CAD build for the part. Positions are in the model's coordinates, mm. A direction names the side the tool comes from. Round coordinates to 2 decimals unless told otherwise and drop trailing zeros. Write each loop counter-clockwise with the first axis right and the second up, starting at its lowest first coordinate (ties: lowest second). Pieces come first, ordered by that corner, then holes. Notation, with made-up numbers: (18, -39) -> (55, -39) arc R16 ccw to (55, -11) -> close; hole circle Ø4 at (43.25, 39). An arc over 180 degrees is marked (long way). Answer in a Markdown table with one row per item. Add a question column.
```python
from build123d import *

# Parameters (mm, degrees)
SKETCH_1_W                   = 30
SKETCH_1_H                   = 35
EXTRUDE_1_DEPTH              = 10.5
CUT_EXTRUDE_1_DEPTH          = 8
FILLET_1_R                   = 1
HOLE_WIZARD_M2_1_D           = 2.1
HOLE_WIZARD_M2_1_DEPTH       = 20
HOLE_WIZARD_M2_1_CBORE_D     = 4.2
HOLE_WIZARD_M2_1_CBORE_DEPTH = 2
HOLE_WIZARD_M2_1_TIP         = 0.63090365


with BuildPart() as part:
    # ｽｹｯﾁ1 → ﾎﾞｽ - 押し出し1 (new body)
    with BuildSketch(Plane(origin=(0, 0, 0), x_dir=(1, 0, 0), z_dir=(0, 1, 0))):
        Rectangle(SKETCH_1_W, SKETCH_1_H)
    extrude(amount=EXTRUDE_1_DEPTH)

    # ｽｹｯﾁ2 → ｶｯﾄ - 押し出し1 (cut)
    with BuildSketch(Plane(origin=(0, 10.5, 0), x_dir=(1, 0, 0), z_dir=(0, 1, 0))):
        with BuildLine():
            Line((15, 12.5), (15, -12.5))
            Line((15, -12.5), (12.5, -12.5))
            ThreePointArc((12.5, -12.5), (10.732233047, -13.232233047), (10, -15))
            Line((10, -15), (10, -17.5))
            Line((10, -17.5), (12.5, -17.5))
            Line((12.5, -17.5), (17, -17.5))
            Line((17, -17.5), (17, 17.5))
            Line((17, 17.5), (12.5, 17.5))
            Line((12.5, 17.5), (10, 17.5))
            Line((10, 17.5), (10, 15))
            ThreePointArc((10, 15), (10.732233047, 13.232233047), (12.5, 12.5))
            Line((12.5, 12.5), (15, 12.5))
        make_face()
    cut_extrude_1 = extrude(amount=-CUT_EXTRUDE_1_DEPTH, mode=Mode.SUBTRACT)

    # ﾐﾗｰ1: ｶｯﾄ - 押し出し1 across plane
    add(cut_extrude_1.mirror(Plane(origin=(0, 0, 0), x_dir=(0, 0, 1), z_dir=(1, 0, 0))), mode=Mode.SUBTRACT)

    # ﾌｨﾚｯﾄ1
    fillet_1_edges = [part.edges().sort_by_distance(p)[0] for p in [
        (15, 10.5, 0),
        (0, 10.5, -17.5),
        (15, 1.25, 17.5),
        (15, 1.25, -17.5),
        (13.75, 10.5, 12.5),
        (10.732233047, 10.5, 13.232233047),
        (10, 10.5, 16.25),
        (13.75, 10.5, -12.5),
        (10, 10.5, -16.25),
        (10.732233047, 10.5, -13.232233047),
        (10, 6.5, -17.5),
        (10, 6.5, 17.5),
        (15, 6.5, 12.5),
        (15, 6.5, -12.5),
        (-15, 10.5, 0),
        (0, 10.5, 17.5),
        (-15, 1.25, 17.5),
        (-15, 1.25, -17.5),
        (-10, 6.5, 17.5),
        (-10.732233047, 10.5, -13.232233047),
        (-13.75, 10.5, -12.5),
        (-15, 6.5, -12.5),
        (-13.75, 10.5, 12.5),
        (-15, 6.5, 12.5),
        (-10.732233047, 10.5, 13.232233047),
        (-10, 10.5, 16.25),
        (-10, 10.5, -16.25),
        (-10, 6.5, -17.5),
    ]]
    fillet(fillet_1_edges, radius=FILLET_1_R)

    # M2 なべ頭ねじ用座ぐり穴1
    with Locations(Plane(origin=(0, 2.5, 0), x_dir=(1, 0, 0), z_dir=(0, 1, 0))):
        with Locations((12.5, -15), (12.5, 15), (-12.5, 15), (-12.5, -15)):
            CounterBoreHole(HOLE_WIZARD_M2_1_D / 2, HOLE_WIZARD_M2_1_CBORE_D / 2, HOLE_WIZARD_M2_1_CBORE_DEPTH, depth=HOLE_WIZARD_M2_1_DEPTH)
            with Locations((0, 0, -(HOLE_WIZARD_M2_1_DEPTH + HOLE_WIZARD_M2_1_TIP / 2))):  # 118° drill point
                Cone(0, HOLE_WIZARD_M2_1_D / 2, HOLE_WIZARD_M2_1_TIP, mode=Mode.SUBTRACT)


solid = part.part
```
Item 1: Pin check, flat tips, straight feed: pin 1 (1.6 mm diameter, centred on y = 6, z = 15.5, fed in from -X); pin 2 (3.5 mm diameter, centred on x = -13, z = 16, fed in from +Y); pin 3 (1.2 mm diameter, centred on x = -13, y = 7, fed in from +Z). Stop position of each tip, or through.
Item 2: Tool access for faces 5 (the cylindrical face through (9.699, 5.951, -17.215)), 6 (the cylindrical face through (9.699, 5.951, 17.215)), 7 (the flat face through (-11.6, 0.5, 15.9)), 8 (the cylindrical face through (-9.699, 5.951, -17.215)): list every direction of +Z, -Z, +X, -X, +Y, -Y with a clear straight run to the whole face (end or side of a thin tool).
Item 3: Saw through at B-B on y = 3.5. Give the cut face in (x, z), then the cut area to 3 significant figures.
Item 4: Drill centre lines: probe 1 along X at (y, z) = (0.35, 15); probe 2 along Z at (x, y) = (-12.5, 0.2); probe 3 along Z at (x, y) = (12.5, 2.05). Where is each one in solid material? Low to high.
Item 5: Saw through at A-A on y = 1. Give the cut face in (x, z).
Item 6: Two-plate mould, pull along Z, no slides. Class faces 1 (the cylindrical face through (12.227, 1.514, 12.918)), 2 (the flat face through (13.4, 0.5, -14.1)), 3 (the cylindrical face through (13.24, 10.215, 12.199)), 4 (the cylindrical face through (9.699, 10.215, -15.74)): +Z half, -Z half, draft (parallel to the pull), parting line (faces both ways), or undercut.
Recorded:
| question | item | result |
|---|---|---|
| 1 | pin 1 | x = -10.02 |
| 1 | pin 2 | y = 2.5 |
| 1 | pin 3 | z = 12.5 |
| 2 | face 5 | -Z, +X, +Y |
| 2 | face 6 | +Z, +X, +Y |
| 2 | face 7 | +Y |
| 2 | face 8 | -Z, -X, +Y |
| 3 | outline | (-15, -11.5) arc R1 ccw to (-14, -12.5) -> (-12.5, -12.5) arc R2.5 cw to (-10, -15) -> (-10, -16.5) arc R1 ccw to (-9, -17.5) -> (9, -17.5) arc R1 ccw to (10, -16.5) -> (10, -15) arc R2.5 cw to (12.5, -12.5) -> (14, -12.5) arc R1 ccw to (15, -11.5) -> (15, 11.5) arc R1 ccw to (14, 12.5) -> (12.5, 12.5) arc R2.5 cw to (10, 15) -> (10, 16.5) arc R1 ccw to (9, 17.5) -> (-9, 17.5) arc R1 ccw to (-10, 16.5) -> (-10, 15) arc R2.5 cw to (-12.5, 12.5) -> (-14, 12.5) arc R1 ccw to (-15, 11.5) -> close |
| 3 | area | 954 mm2 |
| 4 | probe 1 | -15 to -13.55, -11.45 to 11.45, 13.55 to 15 |
| 4 | probe 2 | -17.5 to -16.05, -13.95 to 13.95, 16.05 to 17.5 |
| 4 | probe 3 | -17.5 to -17.1, -12.9 to 12.9, 17.1 to 17.5 |
| 5 | outline | (-15, -16.5) arc R1 ccw to (-14, -17.5) -> (14, -17.5) arc R1 ccw to (15, -16.5) -> (15, 16.5) arc R1 ccw to (14, 17.5) -> (-14, 17.5) arc R1 ccw to (-15, 16.5) -> close; hole circle Ø4.2 at (-12.5, -15); hole circle Ø4.2 at (-12.5, 15); hole circle Ø4.2 at (12.5, -15); hole circle Ø4.2 at (12.5, 15) |
| 6 | face 1 | undercut |
| 6 | face 2 | undercut |
| 6 | face 3 | +Z half |
| 6 | face 4 | draft |
